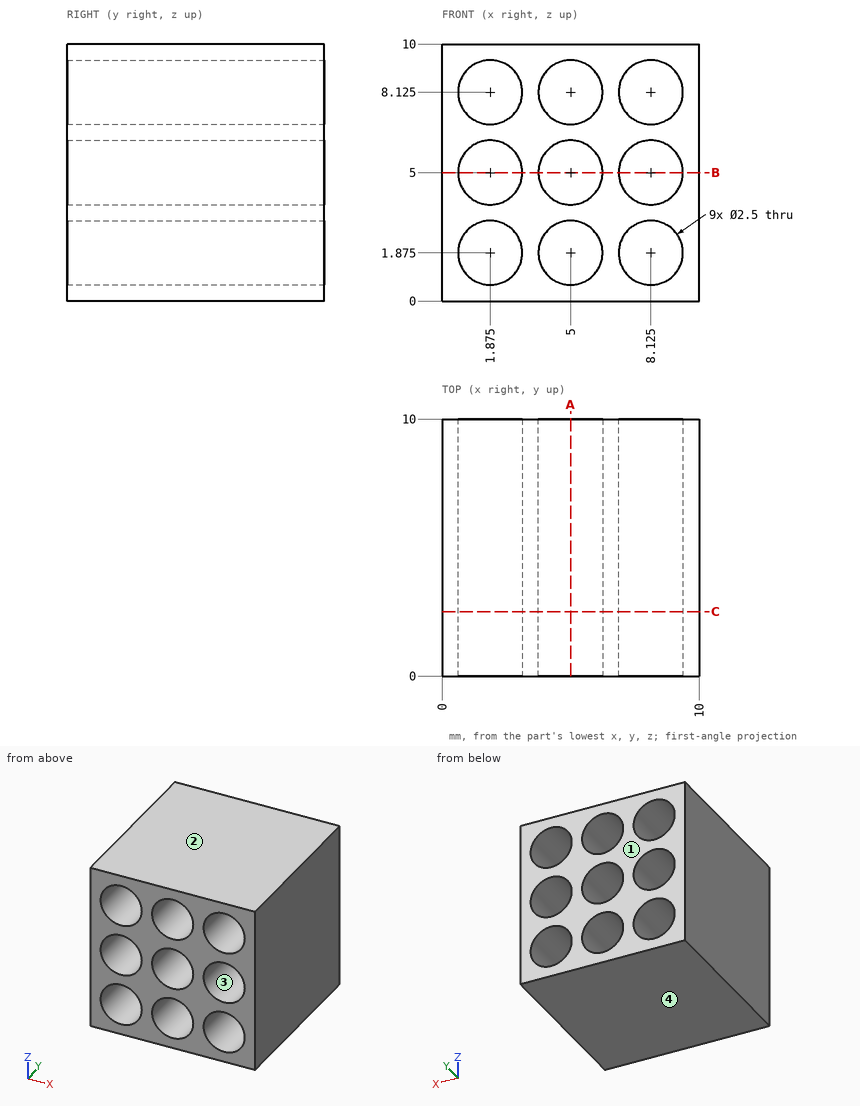
Input: dimensioned drawing with shaded views. Units: mm. Origin: part minimum x, y, z. Coordinates: 2 decimals unless noted, no trailing zeros. Order: outer loops, then holes, each group sorted by start corner. A loop starts at its lowest first (then second) coordinate and runs counter-clockwise, first axis right, second up.
Item 1: Contact query for a flat-ended pin moving along its axis: P1, Ø1.5, axis at x = 1.875, z = 1.875, coming from the +Y side. Output: stop coordinate, or through.
Answer:
P1: passes through
Item 2: Section query B-B (z = 5). Output: boundary loops of the cut face in (x, y) (3 decimals), then the cut area to 3 significant figures.
Answer:
outline: (0, 0) - (0.625, 0) - (0.625, 10) - (0, 10) - close; (3.125, 0) - (3.75, 0) - (3.75, 10) - (3.125, 10) - close; (6.25, 0) - (6.875, 0) - (6.875, 10) - (6.25, 10) - close; (9.375, 0) - (10, 0) - (10, 10) - (9.375, 10) - close
area: 25.0 mm2
Item 3: Section query C-C (y = 2.5). State how many separate pieces and enclosed holes the cut face has, then the cut area to 3 significant figures.
Answer:
separate pieces: 1
enclosed holes: 9
area: 55.8 mm2
Item 4: Section query A-A (x = 5). Output: boundary loops of the cut face in (y, z) (3 decimals), then the cut area to 3 significant figures.
Answer:
outline: (0, 0) - (10, 0) - (10, 0.625) - (0, 0.625) - close; (0, 3.125) - (10, 3.125) - (10, 3.75) - (0, 3.75) - close; (0, 6.25) - (10, 6.25) - (10, 6.875) - (0, 6.875) - close; (0, 9.375) - (10, 9.375) - (10, 10) - (0, 10) - close
area: 25.0 mm2
Item 5: Material intervals for line 1 along Z through (x, y) = (5, 5) (3 decimals); line 2 along Z through (x, y) = (4, 3.75) (3 decimals); line 3 along X through (y, z) = (8.75, 5.75) (3 decimals), sorted ascending.
Answer:
line 1: z = 0 to 0.625, 3.125 to 3.75, 6.25 to 6.875, 9.375 to 10
line 2: z = 0 to 1.125, 2.625 to 4.25, 5.75 to 7.375, 8.875 to 10
line 3: x = 0 to 0.875, 2.875 to 4, 6 to 7.125, 9.125 to 10
Item 6: Draft query along Z for the marked faces 1, 2, 3 and 4. Return one class per face: released by +Z, released by -Z, zero draft, split by the parting line, or undercut.
Answer:
face 1: zero draft
face 2: released by +Z
face 3: undercut
face 4: released by -Z
